Autodesk Inventor part; units mm, degrees
ref_plane "YZ Plane" through (0, 0, 0) normal (1, 0, 0) x (0, 1, 0)
ref_plane "XZ Plane" through (0, 0, 0) normal (0, 1, 0) x (-1, 0, 0)
ref_plane "XY Plane" through (0, 0, 0) normal (0, 0, 1) x (1, 0, 0)
sketch "Sketch1" plane through (0, 0, 0) normal (0, 1, 0) x (-1, 0, 0)
  arc A0 (25.21, 0) -> (-25.21, 0) centre (0, 0) ccw
  arc A1 (27.21, 0) -> (-27.21, 0) centre (0, 0) ccw
  arc A2 (-25.21, -343) -> (25.21, -343) centre (0, -343) ccw
  arc A3 (-27.21, -343) -> (27.21, -343) centre (0, -343) ccw
  line L0 (0, 0) -> (0, -343) construction
  line L1 (27.21, 0) -> (27.21, -343)
  line L2 (-27.21, 0) -> (-27.21, -343)
  line L3 (25.21, 0) -> (25.21, -343)
  line L4 (-25.21, 0) -> (-25.21, -343)
  dimension "d0" = 343
  dimension "d1" = 50.42
  dimension "d2" = 50.42
  dimension "d3" = 2
  dimension "d4" = 2
extrude "Extrusion1" add sketch "Sketch1" along normal blind 6
properties part number "Belt"
Can you work these out from the model? Positions are in its coordinate system, mm. A direction names the side the tool comes from. Give positions to 0.01 mm unless a question says otherwise; leave off trailing zeros. Loops run counter-clockwise (first coordinate to the right, second up) from the corner with the lowest first, then second, coordinate; pieces in that order, holes last. Notation, with made-up numbers: M 19,-3 L 77,-3 A17 cw 77,6 Z; hole C 38,75.25 d2. An arc over 180 degrees is marked long. Answer in a Markdown table with one row per item.
1. Suppose I cut it at A-A on x = 0. Write out the boundary of the cut face in (y, z).
Taken from the geometry:
| item | result |
|---|---|
| outline | M 0,-370.21 L 6,-370.21 L 6,-368.21 L 0,-368.21 Z; M 0,25.21 L 6,25.21 L 6,27.21 L 0,27.21 Z |
2. If I drill on line 1 along Z through (x, y) = (1, 2.95); line 2 along X through (y, z) = (1.75, -321); line 3 along Z through (x, y) = (-5, 5.45), over which ranges is the centre line in solid material (lowest first)?
Taken from the geometry:
| item | result |
|---|---|
| line 1 | z = -370.19 to -368.19, 25.19 to 27.19 |
| line 2 | x = -27.21 to -25.21, 25.21 to 27.21 |
| line 3 | z = -369.75 to -367.71, 24.71 to 26.75 |
3. Thinking about a two-plate mould opening in X: for faces 3 (the cylindrical face through (0.598, 2.958, 27.203)), 4 (the flat face through (-26, 6, -171)), 5 (the cylindrical face through (0.554, 2.958, 25.204)), which applies, released by +X, released by -X, zero draft, split by the parting line, or undercut?
Taken from the geometry:
| item | result |
|---|---|
| face 3 | split by the parting line |
| face 4 | zero draft |
| face 5 | undercut |
4. Suppose I cut it at C-C on z = -291.5. Write out the boundary of the cut face in (x, y), plus the area to 3 significant figures.
Taken from the geometry:
| item | result |
|---|---|
| outline | M -27.21,0 L -25.21,0 L -25.21,6 L -27.21,6 Z; M 25.21,0 L 27.21,0 L 27.21,6 L 25.21,6 Z |
| area | 24.0 mm² |
5. Which directions (+Z, -Z, +X, -X, +Y, -Y) give clear straight access to the entire face, cutting with the end or side of a thin tool? Please do faces 1 (the cylindrical face through (-0.554, 2.958, -368.204)), 2 (the flat face through (-26, 0, -171)).
Taken from the geometry:
| item | result |
|---|---|
| face 1 | +Y, -Y |
| face 2 | +Z, -Z, +X, -X, -Y |
6. Suppose I cut it at B-B on y = 1.65. Write out the boundary of the cut face in (x, z), plus the area to 3 significant figures.
Taken from the geometry:
| item | result |
|---|---|
| outline | M -27.21,-343 A27.21 ccw 27.21,-343 L 27.21,0 A27.21 ccw -27.21,0 Z; hole M -25.21,-343 A25.21 ccw 25.21,-343 L 25.21,0 A25.21 ccw -25.21,0 Z |
| area | 1,700 mm² |
